from build123d import *

# Parameters (mm, degrees)
PAD_DEPTH       = 12
SKETCH001_R     = 2.9
PAD001_DEPTH    = 4.5
SKETCH002_R     = 1.75
POCKET_DEPTH    = 10.501
SKETCH003_R     = 2.2
POCKET001_DEPTH = 5
CHAMFER_SIZE    = 0.5
CHAMFER001_SIZE = 0.5


with BuildPart() as part:
    # Sketch → Pad (new body)
    with BuildSketch(Plane.XY):
        Polygon((-9.125, -4), (-6.125, -4), (-6.125, 0), (6.125, 0), (6.125, -4), (9.125, -4), (9.125, 6), (-9.125, 6), align=None)
    extrude(amount=PAD_DEPTH)

    # Sketch001 (on Face3 of Pad) → Pad001 (join)
    with BuildSketch(Plane.XZ):
        with Locations((0, 6)):
            Circle(SKETCH001_R)
    extrude(amount=PAD001_DEPTH)

    # Sketch002 (on Face12 of Pad001) → Pocket (cut, through all)
    with BuildSketch(Plane.XZ.offset(4.5)):
        with Locations((0, 6)):
            Circle(SKETCH002_R)
    extrude(amount=-POCKET_DEPTH, mode=Mode.SUBTRACT)

    # Sketch003 (on Face6 of Pocket) → Pocket001 (cut)
    with BuildSketch(Plane(origin=(0, 6, 0), x_dir=(-1, 0, 0), z_dir=(0, 1, 0))):
        with Locations((0, 6)):
            Circle(SKETCH003_R)
    extrude(amount=-POCKET001_DEPTH, mode=Mode.SUBTRACT)

    # Chamfer
    chamfer_edges = [part.edges().sort_by_distance(p)[0] for p in [
        (-2.9, -4.5, 6),
    ]]
    chamfer(chamfer_edges, length=CHAMFER_SIZE)

    # Chamfer001
    chamfer001_edges = [part.edges().sort_by_distance(p)[0] for p in [
        (-6.125, -2, 0),
        (-6.125, -2, 12),
        (6.125, -2, 0),
        (9.125, 1, 0),
        (9.125, 1, 12),
        (6.125, -2, 12),
        (-9.125, 1, 12),
        (-9.125, 1, 0),
    ]]
    chamfer(chamfer001_edges, length=CHAMFER001_SIZE)


solid = part.part
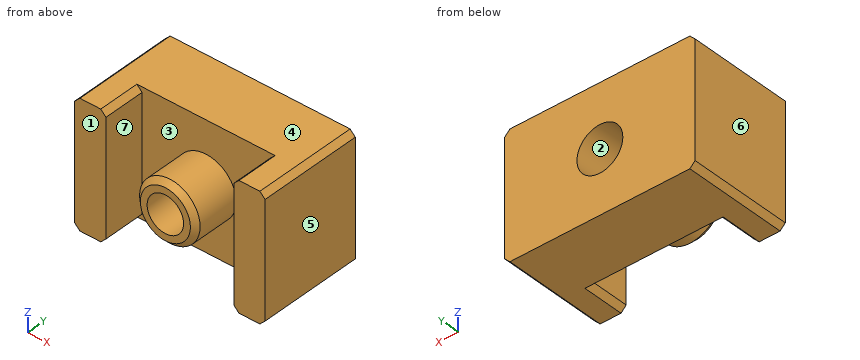
Source: CAD feature listing. Evaluate the final solid. Frame: model axes, mm. Face numbers are marked on the shaded views. A direction names the side the tool comes from. Coordinates: 2 decimals unless noted, no trailing zeros. Loops run counter-clockwise (first coordinate to the right, second up) from the corner with the lowest first, then second, coordinate; pieces in that order, holes last. Notation, with made-up numbers: (47, 53) - (57, 53) arc R37 cw to (57, 92) - close; hole circle Ø7 at (-2.75, 14.25). An arc over 180 degrees is marked (long way). Return JSON: item names as keys, results as strings.
Q1. Contact query for flat-ended pins moving along their axis: P1, Ø3.5, axis at x = -7, z = 4.5, coming from the -Y side; P2, Ø2.5, axis at x = 0, z = 6, coming from the +Y side. Output: stop coordinate, or through.
Results:
{"P1": "y = -4", "P2": "through"}
Q2. Mould query, pull axis X, two halves, no side actions, for the marked faces 4, 5, 6 and 7. Classes: released by +X, released by -X, zero draft, split by the parting line, or undercut.
Results:
{"face 4": "zero draft", "face 5": "released by +X", "face 6": "released by -X", "face 7": "undercut"}
Q3. Section D-D, the plane y = 4.25. Return loops of the section in (x, z) (3 decimals).
Results:
{"outline": "(-9.125, 0.5) - (-8.625, 0) - (8.625, 0) - (9.125, 0.5) - (9.125, 11.5) - (8.625, 12) - (-8.625, 12) - (-9.125, 11.5) - close; hole circle Ø4.4 at (0, 6)"}
Q4. Section B-B, the plane x = 0. Return loops of the section in (y, z).
Results:
{"outline": "(-4.5, 3.6) - (-4, 3.1) - (0, 3.1) - (0, 0) - (6, 0) - (6, 3.8) - (1, 3.8) - (1, 4.25) - (-4.5, 4.25) - close; (-4.5, 7.75) - (1, 7.75) - (1, 8.2) - (6, 8.2) - (6, 12) - (0, 12) - (0, 8.9) - (-4, 8.9) - (-4.5, 8.4) - close"}
Q5. Section C-C, the plane z = 6. Return loops of the section in (x, y) (3 decimals), plus the area to 3 significant figures.
Results:
{"outline": "(-9.125, -4) - (-6.125, -4) - (-6.125, 0) - (-2.9, 0) - (-2.9, -4) - (-2.4, -4.5) - (-1.75, -4.5) - (-1.75, 1) - (-2.2, 1) - (-2.2, 6) - (-9.125, 6) - close; (1.75, -4.5) - (2.4, -4.5) - (2.9, -4) - (2.9, 0) - (6.125, 0) - (6.125, -4) - (9.125, -4) - (9.125, 6) - (2.2, 6) - (2.2, 1) - (1.75, 1) - close", "area": "118 mm2"}
Q6. Section A-A, the plane y = -2. Return loops of the section in (x, z) (3 decimals), plus the area to 3 significant figures.
Results:
{"outline": "(-9.125, 0.5) - (-8.625, 0) - (-6.625, 0) - (-6.125, 0.5) - (-6.125, 11.5) - (-6.625, 12) - (-8.625, 12) - (-9.125, 11.5) - close; circle Ø5.8 at (0, 6); (6.125, 0.5) - (6.625, 0) - (8.625, 0) - (9.125, 0.5) - (9.125, 11.5) - (8.625, 12) - (6.625, 12) - (6.125, 11.5) - close; hole circle Ø3.5 at (0, 6)", "area": "87.8 mm2"}
Q7. Material intervals for line 1 along Z through (x, y) = (0, -0.1); line 2 along Y through (x, z) = (-3.25, 2); line 3 along Y through (x, z) = (8, 11), sorted ascending.
Results:
{"line 1": "3.1 to 4.25, 7.75 to 8.9", "line 2": "0 to 6", "line 3": "-4 to 6"}
Q8. Access query for the marked faces 1, 2 and 3. Directions: +Z, -Z, +X, -X, +Y, -Y. A direction counts if a zero-diameter tool reaches every point of the face in a straight line with its end or side. Return the directions, or none.
Results:
{"face 1": "+Z, -Z, -X, -Y", "face 2": "+Y", "face 3": "-Y"}
